Could you check a few things on this model? Use its own coordinates, in mm. Give positions to 0.01 mm unless a question says otherwise; leave off trailing zeros. Order: outer loops, then holes, each group sorted by start corner. A loop starts at its lowest first (then second) coordinate and runs counter-clockwise, first axis right, second up.
from build123d import *

# Parameters (mm, degrees)
SKETCH2_R           = 1.6637
SKETCH2_W           = 7.62
SKETCH2_H           = 3.81
BOSS_EXTRUDE1_DEPTH = 0.15


with BuildPart() as part:
    # Sketch2 → Boss-Extrude1 (new body)
    with BuildSketch(Plane.XY):
        with BuildLine():
            Line((0, 0), (27.94, 0))
            Line((27.94, 0), (27.94, 13.937675724))
            ThreePointArc((27.94, 13.937675724), (24.7523, 14.605), (27.94, 15.272324276))
            Line((27.94, 15.272324276), (27.94, 34.29))
            Line((27.94, 34.29), (0, 34.29))
            Line((0, 34.29), (0, 15.272324276))
            ThreePointArc((0, 15.272324276), (3.1877, 14.605), (0, 13.937675724))
            Line((0, 13.937675724), (0, 0))
        make_face()
        with Locations((4.445, 22.86)):
            Circle(SKETCH2_R, mode=Mode.SUBTRACT)
        with Locations((4.445, 27.94)):
            Circle(SKETCH2_R, mode=Mode.SUBTRACT)
        with Locations((23.495, 27.94)):
            Circle(SKETCH2_R, mode=Mode.SUBTRACT)
        with Locations((13.97, 27.94)):
            Rectangle(SKETCH2_W, SKETCH2_H, mode=Mode.SUBTRACT)
    extrude(amount=BOSS_EXTRUDE1_DEPTH)


solid = part.part
Item 1: Imagine slicing it at A-A on y = 22.86. List the corners of the cut face in (x, z) for me, then the cut area to 3 significant figures.
Findings:
outline: (0, 0) - (2.78, 0) - (2.78, 0.15) - (0, 0.15) - close; (6.11, 0) - (27.94, 0) - (27.94, 0.15) - (6.11, 0.15) - close
area: 3.69 mm2
Item 2: Please list where these lines run through material, in increasing order: line 1 along Y through (x, z) = (26.25, 0.05); line 2 along X through (y, z) = (27.5, 0.05); line 3 along Y through (x, z) = (14.25, 0.05) (3 decimals).
Findings:
line 1: y = 0 to 12.95, 16.26 to 34.29
line 2: x = 0 to 2.84, 6.05 to 10.16, 17.78 to 21.89, 25.1 to 27.94
line 3: y = 0 to 26.035, 29.845 to 34.29
Item 3: Imagine slicing it at C-C on z = 0.1. List the corners of the cut face in (x, y) for me (3 decimals), then the cut area to 3 significant figures.
Findings:
outline: (0, 0) - (27.94, 0) - (27.94, 13.938) arc R1.664 cw (long way) to (27.94, 15.272) - (27.94, 34.29) - (0, 34.29) - (0, 15.272) arc R1.664 cw (long way) to (0, 13.938) - close; hole circle Ø3.327 at (4.445, 22.86); hole circle Ø3.327 at (4.445, 27.94); hole (10.16, 26.035) - (17.78, 26.035) - (17.78, 29.845) - (10.16, 29.845) - close; hole circle Ø3.327 at (23.495, 27.94)
area: 886 mm2
Item 4: Imagine slicing it at B-B on y = 27.94. List the corners of the cut face in (x, z) for me.
Findings:
outline: (0, 0) - (2.78, 0) - (2.78, 0.15) - (0, 0.15) - close; (6.11, 0) - (10.16, 0) - (10.16, 0.15) - (6.11, 0.15) - close; (17.78, 0) - (21.83, 0) - (21.83, 0.15) - (17.78, 0.15) - close; (25.16, 0) - (27.94, 0) - (27.94, 0.15) - (25.16, 0.15) - close
